```python
from build123d import *

# Parameters (mm, degrees)
PAD_DEPTH            = 20
SKETCH001_W          = 31
SKETCH001_H          = 14
POCKET_DEPTH         = 37.001
POCKET_DEPTH_BACK    = -22.001
SKETCH002_W          = 6
SKETCH002_H          = 2
POCKET001_DEPTH      = 37.001
POCKET001_DEPTH_BACK = -22.001


with BuildPart() as part:
    # Sketch → Pad (new body)
    with BuildSketch(Plane.XY):
        Polygon((-20, 37), (-20, -22), (17, -22), (17, 22), (0, 22), (0, 37), align=None)
    extrude(amount=-PAD_DEPTH)

    # Sketch001 → Pocket (cut, two sides)
    with BuildSketch(Plane.XZ) as pocket_sk:
        with Locations((-4.5, -13)):
            Rectangle(SKETCH001_W, SKETCH001_H)
    extrude(amount=-POCKET_DEPTH, mode=Mode.SUBTRACT)
    extrude(pocket_sk.sketch, amount=-POCKET_DEPTH_BACK, mode=Mode.SUBTRACT)

    # Sketch002 → Pocket001 (cut, two sides)
    with BuildSketch(Plane.XZ) as pocket001_sk:
        with Locations((-3, -1)):
            Rectangle(SKETCH002_W, SKETCH002_H)
    extrude(amount=-POCKET001_DEPTH, mode=Mode.SUBTRACT)
    extrude(pocket001_sk.sketch, amount=-POCKET001_DEPTH_BACK, mode=Mode.SUBTRACT)


solid = part.part
```
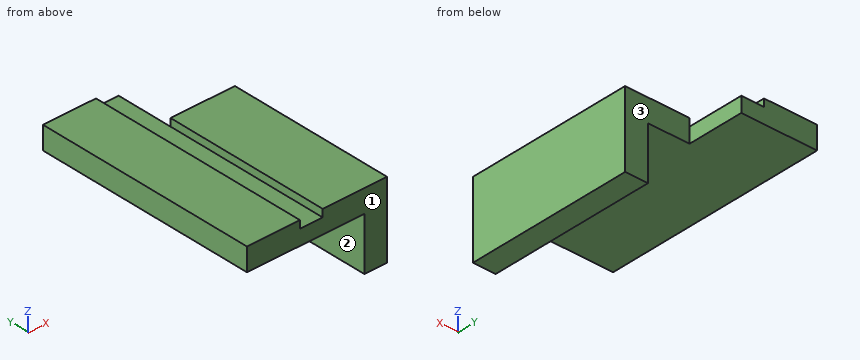
Check sheet for the modelled part. Datum: model origin and axes. Units: mm. Face numbers are marked on the shaded views. A direction names the side the tool comes from. Give positions to 0.01 mm unless a question says otherwise; leave off trailing zeros. Order: outer loops, then holes, each group sorted by start corner. A loop starts at its lowest first (then second) coordinate and runs counter-clockwise, first axis right, second up. Notation, with made-up numbers: (16, -11.75) -> (52, -11.75) arc R20 cw to (52, 18.25) -> close; hole circle Ø11 at (30, 55.25). An arc over 180 degrees is marked (long way). Use CSV: the item, a comma, the result in double quotes. Start each with the question number.
1) Material ranges on line 1 (Z direction, x = 10, y = -11); line 2 (X direction, y = 6, z = -17.75); line 3 (Y direction, x = 4.5, z = -5), recorded low to high. Write a range as from..to.
2) Set-up check for the marked faces 1, 2 and 3: record each of +Z, -Z, +X, -X, +Y, -Y from which the full face is reachable in a straight line by a thin tool's end or side.
3) Go/stop test with flat-tipped pins: P1, Ø4, axis at x = 9.5, z = -17.5, coming from the +Y side; P2, Ø8, axis at x = -14, y = -4.5, coming from the -Z side; P3, Ø8, axis at y = 28.5, z = -6.5, coming from the +X side. Record where each tip stops, or that it passes through.
4) Sectioned sample at C-C, the plane x = -2.5. Record the boundary of the cut face in (y, z), plus the area to 3 significant figures.
5) Sectioned sample at A-A, the plane y = -13.5. Record the boundary of the cut face in (x, z).
6) Sectioned sample at B-B, the plane z = -3.5. Record the boundary of the cut face in (x, y).
7) Sectioned sample at D-D, the plane z = -18.5. Record the boundary of the cut face in (x, y).
Recorded:
1,line 1,"-6..0"
1,line 2,"11..17"
1,line 3,"-22..22"
2,face 1,"+Z, -Z, +X, -X, -Y"
2,face 2,"-Z, -X, +Y, -Y"
2,face 3,"+Z, -Z, +X, +Y"
3,P1,"y = 22"
3,P2,"z = -6"
3,P3,"x = 0"
4,outline,"(-22, -6) -> (37, -6) -> (37, -2) -> (-22, -2) -> close"
4,area,"236 mm2"
5,outline,"(-20, -6) -> (11, -6) -> (11, -20) -> (17, -20) -> (17, 0) -> (0, 0) -> (0, -2) -> (-6, -2) -> (-6, 0) -> (-20, 0) -> close"
6,outline,"(-20, -22) -> (17, -22) -> (17, 22) -> (0, 22) -> (0, 37) -> (-20, 37) -> close"
7,outline,"(11, -22) -> (17, -22) -> (17, 22) -> (11, 22) -> close"
